Verification items for this drawing (mm, ordinates from the low corner). A direction names the side the tool comes from. Give positions to 0.01 mm unless a question says otherwise; leave off trailing zeros. Write each loop counter-clockwise with the first axis right and the second up, starting at its lowest first coordinate (ties: lowest second). Pieces come first, ordered by that corner, then holes. Notation, with made-up numbers: (4, 86.5) -> (55, 86.5) arc R7 cw to (55, 93.5) -> close; hole circle Ø10 at (66.5, 38.5). An arc over 180 degrees is marked (long way). Answer as a JSON object with one key per item and string values.
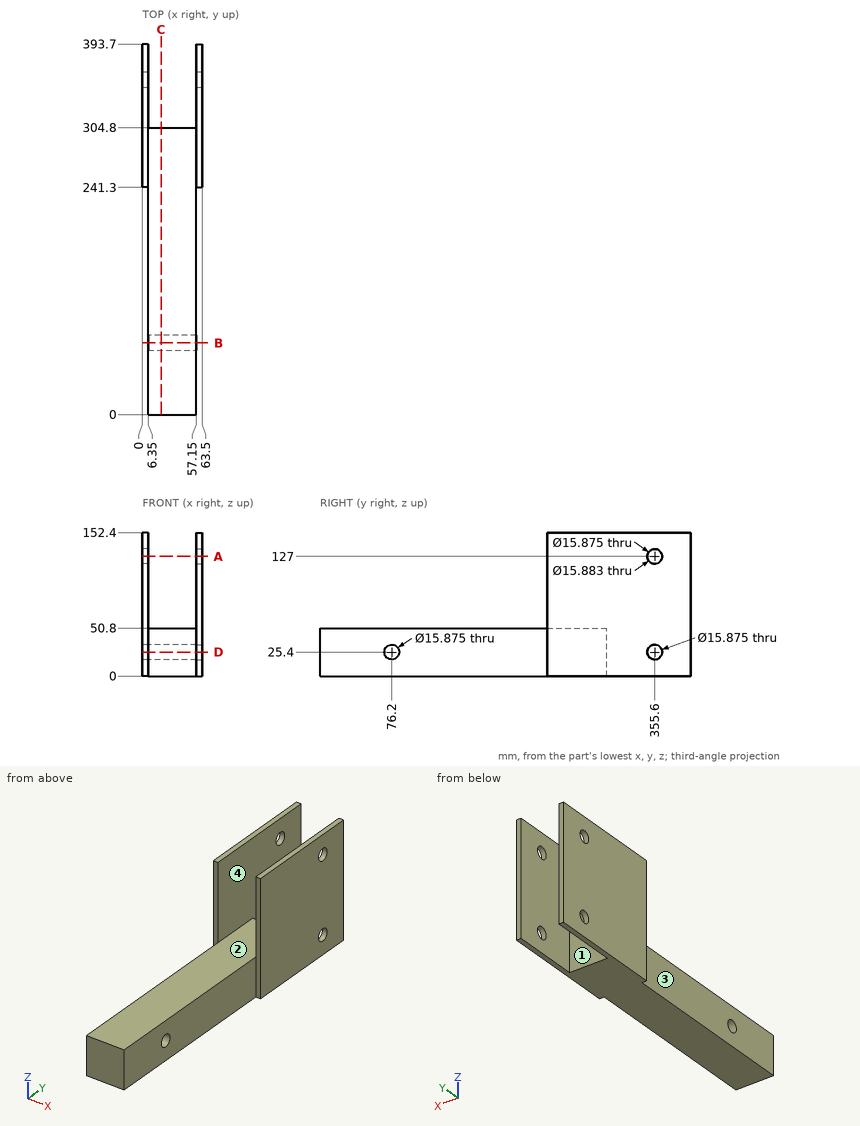
1. Sectioned sample at D-D, the plane z = 25.4. Enter the section's corners in (x, y).
Determined:
{"outline": "(0, 241.3) -> (6.35, 241.3) -> (6.35, 84.14) -> (57.15, 84.14) -> (57.15, 241.3) -> (63.5, 241.3) -> (63.5, 347.66) -> (57.15, 347.66) -> (57.15, 304.8) -> (6.35, 304.8) -> (6.35, 347.66) -> (0, 347.66) -> close; (0, 363.54) -> (6.35, 363.54) -> (6.35, 393.7) -> (0, 393.7) -> close; (6.35, 0) -> (57.15, 0) -> (57.15, 68.26) -> (6.35, 68.26) -> close; (57.15, 363.54) -> (63.5, 363.54) -> (63.5, 393.7) -> (57.15, 393.7) -> close"}
2. Sectioned sample at A-A, the plane z = 127. Enter the section's corners in (x, y).
Determined:
{"outline": "(0, 241.3) -> (6.35, 241.3) -> (6.35, 347.66) -> (0, 347.66) -> close; (0, 363.54) -> (6.35, 363.54) -> (6.35, 393.7) -> (0, 393.7) -> close; (57.15, 241.3) -> (63.5, 241.3) -> (63.5, 347.66) -> (57.15, 347.66) -> close; (57.15, 363.54) -> (63.5, 363.54) -> (63.5, 393.7) -> (57.15, 393.7) -> close"}
3. Access from +Z, -Z, +X, -X, +Y, -Y to the whole of each face (thin tool, end or side, straight path). Record for the marked faces 1, 2, 3 and 4.
Determined:
{"face 1": "+Z, -Z, +Y", "face 2": "+Z, +Y, -Y", "face 3": "+Z, -Z, -X, -Y", "face 4": "+Z, +Y"}
4. Sectioned sample at C-C, the plane x = 20. Enter the section's corners in (y, z) (1 decimal), plus the area to 3 significant figures.
Determined:
{"outline": "(0, 0) -> (304.8, 0) -> (304.8, 50.8) -> (0, 50.8) -> close; hole circle Ø15.9 at (76.2, 25.4)", "area": "15,300 mm^2"}
5. Sectioned sample at B-B, the plane y = 76.2. Enter the section's corners in (x, z).
Determined:
{"outline": "(6.35, 0) -> (57.15, 0) -> (57.15, 17.46) -> (6.35, 17.46) -> close; (6.35, 33.34) -> (57.15, 33.34) -> (57.15, 50.8) -> (6.35, 50.8) -> close"}
6. Scan lines: L1, parallel to X at y = 354, z = 37; L2, parallel to Z at x = 59.5, y = 355.6. Record each from-to range of solid material in increasing order. Write a range as [from, to].
Determined:
{"L1": "[0, 6.35], [57.15, 63.5]", "L2": "[0, 17.46], [33.34, 119.06], [134.94, 152.4]"}
7. Go/stop test with flat-tipped pins: P1, Ø3, axis at x = 2.5, z = 72.5, coming from the -Y side; P2, Ø1, axis at x = 30.5, z = 17.5, coming from the +Y side; P3, Ø6, axis at x = 21.5, y = 260, coming from the +Z side. Record where each tip stops, or that it passes through.
Determined:
{"P1": "y = 241.3", "P2": "y = 304.8", "P3": "z = 50.8"}
